Geometry: see drawing. Coordinates: mm, zero at the bounding-box minimum. Coordinates: 2 decimals unless noted, no trailing zeros. Write each loop counter-clockwise with the first axis right and the second up, starting at its lowest first coordinate (ties: lowest second). Pieces come first, ordered by that corner, then holes.
1) Pin query (flat end, axial travel): pin 1 Ø2 at (x, y) = (20.5, 1) entering from -Z; pin 2 Ø2 at (x, y) = (35, 0.5) entering from -Z. Return the tip coordinate at first contact, or that it passes through.
2) Line query: L1, parallel to X at y = 3.65, z = 26; L2, parallel to X at y = 3.6, z = 14. Output: solid intervals per line, ascending.
3) Section query B-B (z = 26). Output: boundary loops of the cut face in (x, y), then the cut area to 3 significant figures.
4) Section query A-A (x = 26). Output: boundary loops of the cut face in (y, z), then the cut area to 3 significant figures.
5) Section query D-D (x = 7). Output: boundary loops of the cut face in (y, z), then the cut area to 3 significant figures.
6) Section query C-C (y = 1.3). Output: boundary loops of the cut face in (x, z), then the cut area to 3 significant figures.
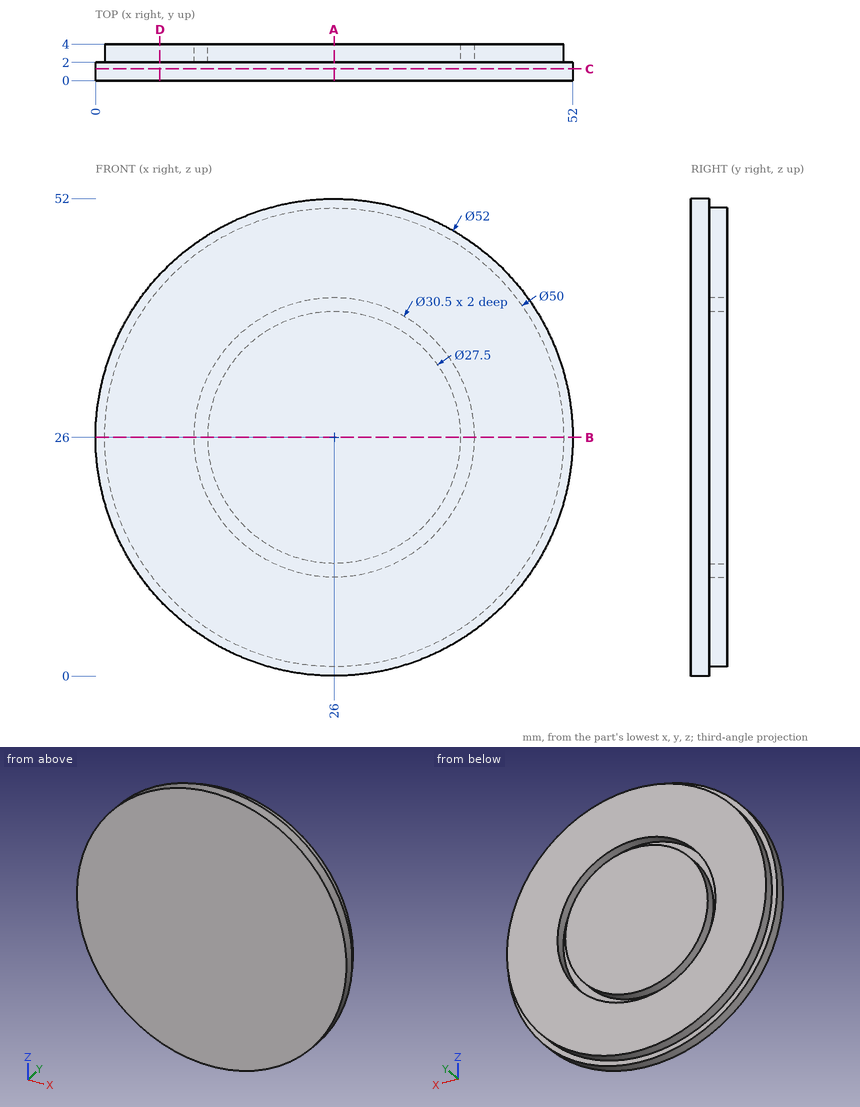
Answer:
1. pin 1: stops at z = 0.39
1. pin 2: stops at z = 1.26
2. L1: x = 1 to 10.75, 12.25 to 39.75, 41.25 to 51
2. L2: x = 4.07 to 16.59, 19.29 to 32.71, 35.41 to 47.93
3. outline: (0, 0) - (52, 0) - (52, 2) - (51, 2) - (51, 4) - (41.25, 4) - (41.25, 2) - (39.75, 2) - (39.75, 4) - (12.25, 4) - (12.25, 2) - (10.75, 2) - (10.75, 4) - (1, 4) - (1, 2) - (0, 2) - close
3. area: 198 mm2
4. outline: (0, 0) - (2, 0) - (2, 1) - (4, 1) - (4, 10.75) - (2, 10.75) - (2, 12.25) - (4, 12.25) - (4, 39.75) - (2, 39.75) - (2, 41.25) - (4, 41.25) - (4, 51) - (2, 51) - (2, 52) - (0, 52) - close
4. area: 198 mm2
5. outline: (0, 8.25) - (2, 8.25) - (2, 9.75) - (4, 9.75) - (4, 42.25) - (2, 42.25) - (2, 43.75) - (0, 43.75) - close
5. area: 136 mm2
6. outline: circle Ø52 at (26, 26)
6. area: 2,120 mm2
